from build123d import *

# Parameters (mm, degrees)
SKETCH1_R                                  = 6.35
BOSS_EXTRUDE1_DEPTH                        = 6.35
SKETCH2_R                                  = 1.7018
CUT_EXTRUDE1_DEPTH                         = 30.648448526
MIRROR1_AT_THE_SECOND_PLANE_COPY_1_SKETC_R = 1.7018
MIRROR1_AT_THE_SECOND_PLANE_COPY_1_DEPTH   = 30.648448526


with BuildPart() as part:
    # Sketch1 → Boss-Extrude1 (new, symmetric)
    with BuildSketch(Plane.XY):
        with BuildLine():
            Line((-12.452586398, 2.494612595), (-13.97, -5.08))
            Line((-13.97, -5.08), (-22.86, -5.08))
            Line((-22.86, -5.08), (-22.86, -12.7))
            Line((-22.86, -12.7), (22.86, -12.7))
            Line((22.86, -12.7), (22.86, -5.08))
            Line((22.86, -5.08), (13.97, -5.08))
            Line((13.97, -5.08), (12.452586398, 2.494612595))
            ThreePointArc((12.452586398, 2.494612595), (0, 12.7), (-12.452586398, 2.494612595))
        make_face()
        Circle(SKETCH1_R, mode=Mode.SUBTRACT)
    extrude(amount=BOSS_EXTRUDE1_DEPTH, both=True)

    # Sketch2 → Cut-Extrude1 (cut, through all)
    with BuildSketch(Plane(origin=(0, -5.08, 0), x_dir=(1, 0, 0), z_dir=(0, 1, 0))):
        with Locations(Location((-19.05, 3.175, 0), (0, 0, 270))):
            Circle(SKETCH2_R)
    cut_extrude1 = extrude(amount=-CUT_EXTRUDE1_DEPTH, mode=Mode.SUBTRACT)

    # Mirror1: Cut-Extrude1 across plane
    add(cut_extrude1.mirror(Plane(origin=(0, 0, 0), x_dir=(0, 0, 1), z_dir=(1, 0, 0))), mode=Mode.SUBTRACT)

    # Mirror1 at the second plane: Cut-Extrude1 across plane
    add(cut_extrude1.mirror(Plane.XY), mode=Mode.SUBTRACT)

    # Mirror1 at the second plane copy 1 sketc → Mirror1 at the second plane copy 1 (cut, through all)
    with BuildSketch(Plane(origin=(0, -5.08, 0), x_dir=(-1, 0, 0), z_dir=(0, 1, 0))):
        with Locations(Location((-19.05, 3.175, 0), (0, 0, 270))):
            Circle(MIRROR1_AT_THE_SECOND_PLANE_COPY_1_SKETC_R)
    extrude(amount=-MIRROR1_AT_THE_SECOND_PLANE_COPY_1_DEPTH, mode=Mode.SUBTRACT)


solid = part.part
Work out the finished part from the listing and answer in its coordinate system (mm). A direction names the side the tool comes from. Coordinates: 2 decimals unless noted, no trailing zeros. Write each loop counter-clockwise with the first axis right and the second up, starting at its lowest first coordinate (ties: lowest second). Pieces come first, ordered by that corner, then holes. Notation, with made-up numbers: M -32,85.5 L 3,85.5 A11 ccw 3,95.5 Z; hole C -18,76 d6. An arc over 180 degrees is marked long. Use one line per item in the form item = value. Start each with the question number.
1. Straight lines are drawn through the part: probe 1 along Z at (x, y) = (19.05, -7.75); probe 2 along X at (y, z) = (-5.75, 2); probe 3 along Y at (x, z) = (19, -0.75). For each, find the intervals that lie inside material, in ascending order. Write a range as from..to.
2. The part is cut by section D-D (z = -0.25). Give the vertices of the cut face in (x, y).
3. The part is cut by section C-C (y = -9.5). Give the vertices of the cut face in (x, z) (3 decimals).
4. The part is cut by section B-B (x = -19.05). Give the vertices of the cut face in (y, z), plus the area to 3 significant figures.
5. A tool of negligible diameter and unlimited length cuts with its end or side. For faces 5 (the face through (22.86, -9, 0)), 6 (the face through (-18, -5.08, 0)), 7 (the face through (18, -5.08, 0)), from which of +Z, -Z, +X, -X, +Y, -Y can it reach the whole face along a straight path? Write none if from no direction.
6. The mould has two halves that part along X. Classify faces 1 (the face through (0, -12.7, 0)), 2 (the face through (0.2, 12.7, 0.1)), 3 (the face through (-1.38, -6.2, -0.09)), 4 (the face through (-13.2, -1.24, 0.09)): released by +X, released by -X, zero draft, split by the parting line, or undercut.
7. The part is cut by section A-A (x = 0). Give the vertices of the cut face in (y, z).
8. Each of these flat-tipped pins is pushed along its axis until it touches: P1, Ø4.5, axis at x = -19.05, z = -3.175, coming from the +Y side; P2, Ø14.5, axis at x = 0, y = 0, coming from the +Z side; P3, Ø5, axis at y = -1, z = 0, coming from the -X side; P4, Ø5, axis at y = 1.5, z = -1.5, coming from the -X side. Where does it stop, or does it pass through?
Evaluation:
q1.probe_1 = -6.35..-4.88, -1.47..1.47, 4.88..6.35
q1.probe_2 = -22.86..-20.28, -17.82..-2.69, 2.69..17.82, 20.28..22.86
q1.probe_3 = -12.7..-5.08
q2.outline = M -22.86,-12.7 L 22.86,-12.7 L 22.86,-5.08 L 13.97,-5.08 L 12.45,2.49 A12.7 ccw -12.45,2.49 L -13.97,-5.08 L -22.86,-5.08 Z; hole C 0,0 d12.7
q3.outline = M -22.86,-6.35 L 22.86,-6.35 L 22.86,6.35 L -22.86,6.35 Z; hole C -19.05,-3.175 d3.404; hole C -19.05,3.175 d3.404; hole C 19.05,-3.175 d3.404; hole C 19.05,3.175 d3.404
q4.outline = M -12.7,-6.35 L -5.08,-6.35 L -5.08,-4.88 L -12.7,-4.88 Z; M -12.7,-1.47 L -5.08,-1.47 L -5.08,1.47 L -12.7,1.47 Z; M -12.7,4.88 L -5.08,4.88 L -5.08,6.35 L -12.7,6.35 Z
q4.area = 44.9 mm^2
q5.face_5 = +Z, -Z, +X, +Y, -Y
q5.face_6 = +Z, -Z, -X, +Y
q5.face_7 = +Z, -Z, +X, +Y
q6.face_1 = zero draft
q6.face_2 = split by the parting line
q6.face_3 = undercut
q6.face_4 = released by -X
q7.outline = M -12.7,-6.35 L -6.35,-6.35 L -6.35,6.35 L -12.7,6.35 Z; M 6.35,-6.35 L 12.7,-6.35 L 12.7,6.35 L 6.35,6.35 Z
q8.P1 = -5.08
q8.P2 = 6.35
q8.P3 = -13.65
q8.P4 = -13.15
